from build123d import *

# Parameters (mm, degrees)
F1_R     = 3.6500000581
F1_R_2   = 3.3500010893
F1_R_3   = 3.649998717
F1_R_4   = 1.65
F1_R_5   = 1.35
F2_DEPTH = 2
F3_DEPTH = 25
F4_DEPTH = 23
F5_R     = 2


with BuildPart() as f2:
    # F1 (on Top) → F2 (new body)
    with BuildSketch(Plane.XY):
        with BuildLine():
            Line((42.8394566104, 17.9592743516), (-22.1605433896, 17.9592743516))
            ThreePointArc((-22.1605433896, 17.9592743516), (-27.1102905971, 15.909021928), (-29.1605430207, 10.9592747205))
            Line((-29.1605430207, 10.9592747205), (-29.1605430207, -29.0407252795))
            ThreePointArc((-29.1605430207, -29.0407252795), (-27.1102905971, -33.9904724869), (-22.1605433896, -36.0407249106))
            Line((-22.1605433896, -36.0407249106), (42.8394566104, -36.0407249106))
            ThreePointArc((42.8394566104, -36.0407249106), (47.7892038178, -33.9904724869), (49.8394562415, -29.0407252795))
            Line((49.8394562415, -29.0407252795), (49.8394562415, 10.9592747205))
            ThreePointArc((49.8394562415, 10.9592747205), (47.7892038178, 15.909021928), (42.8394566104, 17.9592743516))
        make_face()
        with BuildLine():
            ThreePointArc((-27.1605433896, 10.9592747205), (-25.6960772956, 14.4948086265), (-22.1605433896, 15.9592747205))
            Line((-22.1605433896, 15.9592747205), (42.8394566104, 15.9592747205))
            ThreePointArc((42.8394566104, 15.9592747205), (46.3749905163, 14.4948086265), (47.8394566104, 10.9592747205))
            Line((47.8394566104, 10.9592747205), (47.8394566104, -29.0407252795))
            ThreePointArc((47.8394566104, -29.0407252795), (46.3749905163, -32.5762591854), (42.8394566104, -34.0407252795))
            Line((42.8394566104, -34.0407252795), (-22.1605433896, -34.0407252795))
            ThreePointArc((-22.1605433896, -34.0407252795), (-25.6960772956, -32.5762591854), (-27.1605433896, -29.0407252795))
            Line((-27.1605433896, -29.0407252795), (-27.1605433896, 10.9592747205))
        make_face(mode=Mode.SUBTRACT)
        with BuildLine():
            Line((42.8394566104, 15.9592747205), (-22.1605433896, 15.9592747205))
            ThreePointArc((-22.1605433896, 15.9592747205), (-25.6960772956, 14.4948086265), (-27.1605433896, 10.9592747205))
            Line((-27.1605433896, 10.9592747205), (-27.1605433896, -29.0407252795))
            ThreePointArc((-27.1605433896, -29.0407252795), (-25.6960772956, -32.5762591854), (-22.1605433896, -34.0407252795))
            Line((-22.1605433896, -34.0407252795), (42.8394566104, -34.0407252795))
            ThreePointArc((42.8394566104, -34.0407252795), (46.3749905163, -32.5762591854), (47.8394566104, -29.0407252795))
            Line((47.8394566104, -29.0407252795), (47.8394566104, 10.9592747205))
            ThreePointArc((47.8394566104, 10.9592747205), (46.3749905163, 14.4948086265), (42.8394566104, 15.9592747205))
        make_face()
        with Locations((-22.1605433896, -29.0407252795)):
            Circle(F1_R, mode=Mode.SUBTRACT)
        with Locations((42.8394566104, -29.0407252795)):
            Circle(F1_R_2, mode=Mode.SUBTRACT)
        with Locations((-22.1605433896, 10.9592747205)):
            Circle(F1_R, mode=Mode.SUBTRACT)
        with Locations((42.8394566104, 10.9592747205)):
            Circle(F1_R_3, mode=Mode.SUBTRACT)
        with Locations((-22.1605433896, 10.9592747205)):
            Circle(F1_R)
        with Locations((-22.1605433896, 10.9592747205)):
            Circle(F1_R_4, mode=Mode.SUBTRACT)
        with Locations((-22.1605433896, -29.0407252795)):
            Circle(F1_R)
        with Locations((-22.1605433896, -29.0407252795)):
            Circle(F1_R_4, mode=Mode.SUBTRACT)
        with Locations((42.8394566104, 10.9592747205)):
            Circle(F1_R_3)
        with Locations((42.8394566104, 10.9592747205)):
            Circle(F1_R_4, mode=Mode.SUBTRACT)
        with Locations((42.8394566104, -29.0407252795)):
            Circle(F1_R_2)
        with Locations((42.8394566104, -29.0407252795)):
            Circle(F1_R_5, mode=Mode.SUBTRACT)
        with Locations((42.8394566104, 10.9592747205)):
            Circle(F1_R_4)
        with Locations((-22.1605433896, 10.9592747205)):
            Circle(F1_R_4)
        with Locations((-22.1605433896, -29.0407252795)):
            Circle(F1_R_4)
        with Locations((42.8394566104, -29.0407252795)):
            Circle(F1_R_5)
    extrude(amount=F2_DEPTH)

    # F1 (on Top) → F3 (join)
    with BuildSketch(Plane.XY):
        with BuildLine():
            Line((42.8394566104, 17.9592743516), (-22.1605433896, 17.9592743516))
            ThreePointArc((-22.1605433896, 17.9592743516), (-27.1102905971, 15.909021928), (-29.1605430207, 10.9592747205))
            Line((-29.1605430207, 10.9592747205), (-29.1605430207, -29.0407252795))
            ThreePointArc((-29.1605430207, -29.0407252795), (-27.1102905971, -33.9904724869), (-22.1605433896, -36.0407249106))
            Line((-22.1605433896, -36.0407249106), (42.8394566104, -36.0407249106))
            ThreePointArc((42.8394566104, -36.0407249106), (47.7892038178, -33.9904724869), (49.8394562415, -29.0407252795))
            Line((49.8394562415, -29.0407252795), (49.8394562415, 10.9592747205))
            ThreePointArc((49.8394562415, 10.9592747205), (47.7892038178, 15.909021928), (42.8394566104, 17.9592743516))
        make_face()
        with BuildLine():
            ThreePointArc((-27.1605433896, 10.9592747205), (-25.6960772956, 14.4948086265), (-22.1605433896, 15.9592747205))
            Line((-22.1605433896, 15.9592747205), (42.8394566104, 15.9592747205))
            ThreePointArc((42.8394566104, 15.9592747205), (46.3749905163, 14.4948086265), (47.8394566104, 10.9592747205))
            Line((47.8394566104, 10.9592747205), (47.8394566104, -29.0407252795))
            ThreePointArc((47.8394566104, -29.0407252795), (46.3749905163, -32.5762591854), (42.8394566104, -34.0407252795))
            Line((42.8394566104, -34.0407252795), (-22.1605433896, -34.0407252795))
            ThreePointArc((-22.1605433896, -34.0407252795), (-25.6960772956, -32.5762591854), (-27.1605433896, -29.0407252795))
            Line((-27.1605433896, -29.0407252795), (-27.1605433896, 10.9592747205))
        make_face(mode=Mode.SUBTRACT)
    extrude(amount=F3_DEPTH)

    # F1 (on Top) → F4 (join)
    with BuildSketch(Plane.XY):
        with Locations((42.8394566104, 10.9592747205)):
            Circle(F1_R_3)
        with Locations((42.8394566104, 10.9592747205)):
            Circle(F1_R_4, mode=Mode.SUBTRACT)
        with Locations((42.8394566104, -29.0407252795)):
            Circle(F1_R_2)
        with Locations((42.8394566104, -29.0407252795)):
            Circle(F1_R_5, mode=Mode.SUBTRACT)
        with Locations((-22.1605433896, 10.9592747205)):
            Circle(F1_R)
        with Locations((-22.1605433896, 10.9592747205)):
            Circle(F1_R_4, mode=Mode.SUBTRACT)
        with Locations((-22.1605433896, -29.0407252795)):
            Circle(F1_R)
        with Locations((-22.1605433896, -29.0407252795)):
            Circle(F1_R_4, mode=Mode.SUBTRACT)
    extrude(amount=F4_DEPTH)

    # F5
    f5_edges = [f2.edges().sort_by_distance(p)[0] for p in [
        (10.339457, -36.040725, 0),
    ]]
    fillet(f5_edges, radius=F5_R)


solid = f2.part
CAD build for the part. Positions are in the model's coordinates, mm. A direction names the side the tool comes from. Round coordinates to 2 decimals unless told otherwise and drop trailing zeros. Loops run counter-clockwise (first coordinate to the right, second up) from the corner with the lowest first, then second, coordinate; pieces in that order, holes last.
(1) Cut at C-C (x = 7.5). Give the cut face in (y, z).
(2) Which spindle directions (+Z, -Z, +X, -X, +Y, -Y) get a long thin tool onto all of the face, cutting with end or side? Do faces 1 (the flat face through (47.839, -9, 13)), 2 (the flat face through (11, 17.959, 13)). Say none if no direction does.
(3) Cut at A-A (z = 15.5). State how many separate pieces and enclosed holes the cut face has, plus the area to 3 significant figures.
(4) Cut at B-B (y = -9.5). Give the cut face in (x, z), plus the area to 3 significant figures.
(5) Drop flat-ended pins along their axis: pin 1 (2.5 mm diameter, centred on x = -22.16, y = -29.04, fed in from +Z); pin 2 (2.5 mm diameter, centred on x = 42.5, y = 10.5, fed in from +Z). Give the stop position or say it passes through.
(6) Wall check: line 1 along X through (y, z) = (11, 8.5); line 2 along X through (y, z) = (4.5, 3.75); line 3 along Y through (x, z) = (5, 5.5). Give the ranges that are in metal, low to high.
Findings below:
1. outline: (-36.04, 2) arc R2 ccw to (-34.04, 0) - (15.96, 0) arc R2 ccw to (17.96, 2) - (17.96, 25) - (15.96, 25) - (15.96, 2) - (-34.04, 2) - (-34.04, 25) - (-36.04, 25) - close
2. face 1: +Z
2. face 2: +Z, -Z, +X, -X, +Y
3. separate pieces: 5
3. enclosed holes: 5
3. area: 625 mm2
4. outline: (-29.16, 2) arc R2 ccw to (-27.16, 0) - (47.84, 0) arc R2 ccw to (49.84, 2) - (49.84, 25) - (47.84, 25) - (47.84, 2) - (-27.16, 2) - (-27.16, 25) - (-29.16, 25) - close
4. area: 248 mm2
5. pin 1: stops at z = 2
5. pin 2: stops at z = 23
6. line 1: x = -29.16 to -27.16, -25.81 to -23.81, -20.51 to -18.51, 39.19 to 41.19, 44.49 to 46.49, 47.84 to 49.84
6. line 2: x = -29.16 to -27.16, 47.84 to 49.84
6. line 3: y = -36.04 to -34.04, 15.96 to 17.96
